```python
from build123d import *

# Parameters (mm, degrees)
REVOLVE1_ANGLE     = 180
CUT_REVOLVE1_ANGLE = 180
SKETCH3_R          = 10
CUT_EXTRUDE1_DEPTH = 362


with BuildPart() as part:
    # Sketch1 → Revolve1 (revolve)
    with BuildSketch(Plane.XY):
        with BuildLine():
            Line((0, 215), (0, -215))
            ThreePointArc((0, -215), (215, 0), (0, 215))
        make_face()
    revolve(axis=Axis((0, 215, 0), (0, -1, 0)), revolution_arc=REVOLVE1_ANGLE)

    # Sketch2 → Cut-Revolve1 (revolve, cut)
    with BuildSketch(Plane(origin=(0, 0, 0), x_dir=(-1, 0, 0), z_dir=(0, 0, -1))):
        with BuildLine():
            Line((0, 205), (0, -205))
            ThreePointArc((0, -205), (205, 0), (0, 205))
        make_face()
    revolve(axis=Axis((0, 205, 0), (0, 1, 0)), revolution_arc=CUT_REVOLVE1_ANGLE, mode=Mode.SUBTRACT)

    # Sketch3 → Cut-Extrude1 (cut)
    with BuildSketch(Plane.XY):
        with Locations(Location((0, 0, 0), (0, 0, 180))):
            Circle(SKETCH3_R)
    extrude(amount=CUT_EXTRUDE1_DEPTH, mode=Mode.SUBTRACT)


solid = part.part
```
The model under review builds one solid part; all positions refer to its coordinate system, in mm. Round coordinates to 2 decimals unless told otherwise and drop trailing zeros. Order: outer loops, then holes, each group sorted by start corner. A loop starts at its lowest first (then second) coordinate and runs counter-clockwise, first axis right, second up. Notation, with made-up numbers: (30, 10.5) -> (89, 10.5) arc R13 cw to (89, 18.5) -> close; hole circle Ø3 at (16.25, 29.5). An arc over 180 degrees is marked (long way). One line per item, written item: value. Start each with the question number.
Q1. Take a section at C-C (z = 53.5). Write out the cut boundary in (x, y).
Q2. Take a section at A-A (x = 0). Write out the cut boundary in (y, z).
Q3. Clearance check with flat-ended pins moving along their axes: pin 1 Ø2 at (x, z) = (-34, 188) entering from +Y; pin 2 Ø10 at (x, z) = (94, 115.5) entering from -Y; pin 3 Ø10 at (x, y) = (26, -74) entering from +Z. State where each tip first meets the part, or that it passes through.
Q4. Mouldability with a two-part tool opening along X and no side actions: class faces 1 (the face through (190, -79, 0)), 2 (the face through (10, 0, 210)) as released by +X, released by -X, zero draft, split by the parting line, or undercut.
Q5. Wall thickness on line 1 (Y direction, x = 101.5, z = 158.5); line 2 (X direction, y = 127.5, z = 21); line 3 (X direction, y = -6, z = 179.5): over which ranges is each line inside the solid? List them lowest first.
Reported:
1. outline: circle Ø416.47 at (0, 0); hole circle Ø395.79 at (0, 0)
2. outline: (-215, 0) -> (-205, 0) arc R205 cw to (-10, 204.76) -> (-10, 214.77) arc R215 ccw to start; (10, 204.76) arc R205 cw to (205, 0) -> (215, 0) arc R215 ccw to (10, 214.77) -> close
3. pin 1: stops at y = 100.53
3. pin 2: stops at y = -159.73
3. pin 3: stops at z = 202.07
4. face 1: zero draft
4. face 2: undercut
5. line 1: y = -103.93 to -81.24, 81.24 to 103.93
5. line 2: x = -171.84 to -159.15, 159.15 to 171.84
5. line 3: x = -118.19 to -98.84, 98.84 to 118.19
